from build123d import *

# Parameters (mm, degrees)
SKETCH1_W           = 203.2
SKETCH1_H           = 127
BOSS_EXTRUDE1_DEPTH = 44.45
SKETCH2_W           = 196.85
SKETCH2_H           = 120.65
CUT_EXTRUDE1_DEPTH  = 45.45
SKETCH4_W           = 203.2
SKETCH4_H           = 127
SKETCH4_W_2         = 196.85
SKETCH4_H_2         = 120.65
BOSS_EXTRUDE2_DEPTH = 6.35
CUT_EXTRUDE5_DEPTH  = 128
CUT_EXTRUDE6_REACH  = 205.2
CUT_EXTRUDE7_REACH  = 205.2
SKETCH13_R          = 12.55395


with BuildPart() as part:
    # Sketch1 → Boss-Extrude1 (new body)
    with BuildSketch(Plane(origin=(0, 0, 0), x_dir=(1, 0, 0), z_dir=(0, 1, 0))):
        Rectangle(SKETCH1_W, SKETCH1_H)
    extrude(amount=BOSS_EXTRUDE1_DEPTH)

    # Sketch2 → Cut-Extrude1 (cut, through all)
    with BuildSketch(Plane(origin=(0, 44.45, 0), x_dir=(1, 0, 0), z_dir=(0, 1, 0))):
        Rectangle(SKETCH2_W, SKETCH2_H)
    extrude(amount=-CUT_EXTRUDE1_DEPTH, mode=Mode.SUBTRACT)

    # Sketch4 → Boss-Extrude2 (add)
    with BuildSketch(Plane(origin=(0, 44.45, 0), x_dir=(1, 0, 0), z_dir=(0, 1, 0))):
        Rectangle(SKETCH4_W, SKETCH4_H)
        Rectangle(SKETCH4_W_2, SKETCH4_H_2, mode=Mode.SUBTRACT)
    extrude(amount=-BOSS_EXTRUDE2_DEPTH)

    # Sketch10 → Cut-Extrude5 (cut, through all)
    with BuildSketch(Plane.XY.offset(63.5)):
        with BuildLine():
            ThreePointArc((-65.9511, 22.225), (-81.206975571, 31.167602912), (-81.556705839, 13.4874))
            Line((-81.556705839, 13.4874), (-70.843294161, 13.4874))
            ThreePointArc((-70.843294161, 13.4874), (-67.257397088, 17.218024429), (-65.9511, 22.225))
        make_face()
        with BuildLine():
            ThreePointArc((-15.1511, 22.225), (-30.406975571, 31.167602912), (-30.756705839, 13.4874))
            Line((-30.756705839, 13.4874), (-20.043294161, 13.4874))
            ThreePointArc((-20.043294161, 13.4874), (-16.457397088, 17.218024429), (-15.1511, 22.225))
        make_face()
        with BuildLine():
            ThreePointArc((35.6489, 22.225), (20.393024429, 31.167602912), (20.043294161, 13.4874))
            Line((20.043294161, 13.4874), (30.756705839, 13.4874))
            ThreePointArc((30.756705839, 13.4874), (34.342602912, 17.218024429), (35.6489, 22.225))
        make_face()
        with BuildLine():
            Line((70.843294161, 13.4874), (81.556705839, 13.4874))
            ThreePointArc((81.556705839, 13.4874), (85.142602912, 17.218024429), (86.4489, 22.225))
            ThreePointArc((86.4489, 22.225), (71.193024429, 31.167602912), (70.843294161, 13.4874))
        make_face()
    extrude(amount=-CUT_EXTRUDE5_DEPTH, mode=Mode.SUBTRACT)

    # Sketch12 → Cut-Extrude6 (cut, up to next)
    with BuildSketch(Plane(origin=(101.6, 0, 0), x_dir=(0, 0, -1), z_dir=(1, 0, 0)), mode=Mode.PRIVATE) as cut_extrude6_sk1:
        with BuildLine():
            ThreePointArc((-20.043294161, 13.4874), (-25.4, 32.4739), (-30.756705839, 13.4874))
            Line((-30.756705839, 13.4874), (-20.043294161, 13.4874))
        make_face()
    cut_extrude6_tool1 = extrude(cut_extrude6_sk1.sketch, amount=-CUT_EXTRUDE6_REACH, mode=Mode.PRIVATE) & part.part
    add(cut_extrude6_tool1.solids().sort_by_distance((101.6, 22.546198, 25.4))[0], mode=Mode.SUBTRACT)
    # Sketch12 → Cut-Extrude6 (cut, up to next)
    with BuildSketch(Plane(origin=(101.6, 0, 0), x_dir=(0, 0, -1), z_dir=(1, 0, 0)), mode=Mode.PRIVATE) as cut_extrude6_sk2:
        with BuildLine():
            ThreePointArc((30.756705839, 13.4874), (25.4, 32.4739), (20.043294161, 13.4874))
            Line((20.043294161, 13.4874), (30.756705839, 13.4874))
        make_face()
    cut_extrude6_tool2 = extrude(cut_extrude6_sk2.sketch, amount=-CUT_EXTRUDE6_REACH, mode=Mode.PRIVATE) & part.part
    add(cut_extrude6_tool2.solids().sort_by_distance((101.6, 22.546198, -25.4))[0], mode=Mode.SUBTRACT)

    # Sketch13 → Cut-Extrude7 (cut, up to next)
    with BuildSketch(Plane.ZY.offset(101.6), mode=Mode.PRIVATE) as cut_extrude7_sk1:
        with Locations((12.7, 22.225)):
            Circle(SKETCH13_R)
    cut_extrude7_tool1 = extrude(cut_extrude7_sk1.sketch, amount=-CUT_EXTRUDE7_REACH, mode=Mode.PRIVATE) & part.part
    add(cut_extrude7_tool1.solids().sort_by_distance((-101.6, 22.225, 12.7))[0], mode=Mode.SUBTRACT)


solid = part.part
Input: part model. Units: mm. Frame: model coordinates. A direction names the side the tool comes from. Coordinates: 2 decimals unless noted, no trailing zeros. Loops run counter-clockwise (first coordinate to the right, second up) from the corner with the lowest first, then second, coordinate; pieces in that order, holes last. Notation, with made-up numbers: (-22.75, 80.25) -> (-3.75, 80.25) arc R12 ccw to (-3.75, 91.25) -> close; hole circle Ø7 at (33.5, 6). An arc over 180 degrees is marked (long way). One line per item, written item: value.
(1) Cut plane A-A (z = 50). Output: boundary loops of the cut face in (x, y) (3 decimals), then the cut area to 3 significant figures.
Answer below:
outline: (-101.6, 0) -> (-98.425, 0) -> (-98.425, 44.45) -> (-101.6, 44.45) -> close; (98.425, 0) -> (101.6, 0) -> (101.6, 44.45) -> (98.425, 44.45) -> close
area: 282 mm2
(2) Ray query, line 1 along Z through (x, y) = (-14, 31.5) (3 decimals); line 2 along Y through (x, z) = (-76.2, 61.3); line 3 along X through (y, z) = (20.5, -8.5) (3 decimals). Return the intervals inside material, ascending.
Answer below:
line 1: z = -63.5 to -60.325, 60.325 to 63.5
line 2: y = 0 to 13.49, 32.47 to 44.45
line 3: x = -101.6 to -98.425, 98.425 to 101.6
(3) Set-up query: faces 1 (the face through (-1, 23, 60.325)), 2 (the face through (-1, 22, 63.5)), 3 (the face through (-100.03, 22.78, 0.16)), 4 (the face through (-101.6, 17, 1)), 5 (the face through (100.035, 32.467, 25.028)). Return all of +Z, -Z, +X, -X, +Y, -Y with unobstructed straight access to the full face (end or side cutting, diameter ignored); none if empty.
Answer below:
face 1: +Y, -Y
face 2: +Z, +X, -X, +Y, -Y
face 3: -X
face 4: +Z, -Z, -X, +Y, -Y
face 5: +X
(4) Cut plane C-C (x = -76.2). Output: boundary loops of the cut face in (y, z) (3 decimals).
Answer below:
outline: (0, -63.5) -> (13.487, -63.5) -> (13.487, -60.325) -> (0, -60.325) -> close; (0, 60.325) -> (13.487, 60.325) -> (13.487, 63.5) -> (0, 63.5) -> close; (32.474, -63.5) -> (44.45, -63.5) -> (44.45, -60.325) -> (32.474, -60.325) -> close; (32.474, 60.325) -> (44.45, 60.325) -> (44.45, 63.5) -> (32.474, 63.5) -> close
(5) Cut plane B-B (x = 6.5). Output: boundary loops of the cut face in (y, z) (3 decimals), then the cut area to 3 significant figures.
Answer below:
outline: (0, -63.5) -> (44.45, -63.5) -> (44.45, -60.325) -> (0, -60.325) -> close; (0, 60.325) -> (44.45, 60.325) -> (44.45, 63.5) -> (0, 63.5) -> close
area: 282 mm2
(6) Cut plane D-D (y = 41.5). Output: boundary loops of the cut face in (x, z) (3 decimals).
Answer below:
outline: (-101.6, -63.5) -> (101.6, -63.5) -> (101.6, 63.5) -> (-101.6, 63.5) -> close; hole (-98.425, -60.325) -> (98.425, -60.325) -> (98.425, 60.325) -> (-98.425, 60.325) -> close
(7) Draft query along X for faces 6 (the face through (100.035, 32.467, -25.772)), 7 (the face through (-1, 23, -60.325)), 8 (the face through (101.6, 22, 1)). Return one class per face: pulls with the +X half, pulls with the -X half, needs draft (parallel to the pull), parting line crosses it, or undercut.
Answer below:
face 6: needs draft
face 7: undercut
face 8: pulls with the +X half
